Read the model definition and answer for the solid it produces. Units are mm, in the model's axes. Face numbers are marked on the shaded views. Coordinates: 2 decimals unless noted, no trailing zeros. Order: outer loops, then holes, each group sorted by start corner. A loop starts at its lowest first (then second) coordinate and runs counter-clockwise, first axis right, second up. Notation, with made-up numbers: (-25, 45) -> (-15, 45) arc R28 ccw to (-15, 71) -> close; hole circle Ø3 at (14, -8.5). An arc over 180 degrees is marked (long way). Use CSV: the item, a comma, the result in double quotes.
```python
from build123d import *

# Parameters (mm, degrees)
SKETCH1_R           = 32
SKETCH1_R_2         = 2
SKETCH1_R_3         = 4
BOSS_EXTRUDE1_DEPTH = 3
FILLET1_R           = 50


with BuildPart() as part:
    # Sketch1 → Boss-Extrude1 (new body)
    with BuildSketch(Plane(origin=(0, 0, 0), x_dir=(1, 0, 0), z_dir=(0, 1, 0))):
        with Locations(Location((0, 0, 0), (0, 0, 270))):
            Circle(SKETCH1_R)
        with Locations(Location((0, 10, 0), (0, 0, 270))):
            Circle(SKETCH1_R_2, mode=Mode.SUBTRACT)
        with Locations(Location((0, -5, 0), (0, 0, 270))):
            Circle(SKETCH1_R_2, mode=Mode.SUBTRACT)
        with Locations(Location((0, 21.162401824, 0), (0, 0, 270))):
            Circle(SKETCH1_R_3, mode=Mode.SUBTRACT)
        with Locations(Location((16.54543199, 13.19454172, 0), (0, 0, 270))):
            Circle(SKETCH1_R_3, mode=Mode.SUBTRACT)
        with Locations(Location((20.631816227, -4.709077419, 0), (0, 0, 270))):
            Circle(SKETCH1_R_3, mode=Mode.SUBTRACT)
        with Locations(Location((9.182022032, -19.066665213, 0), (0, 0, 270))):
            Circle(SKETCH1_R_3, mode=Mode.SUBTRACT)
        with Locations(Location((-9.182022032, -19.066665213, 0), (0, 0, 270))):
            Circle(SKETCH1_R_3, mode=Mode.SUBTRACT)
        with Locations(Location((-20.631816227, -4.709077419, 0), (0, 0, 270))):
            Circle(SKETCH1_R_3, mode=Mode.SUBTRACT)
        with Locations(Location((-16.54543199, 13.19454172, 0), (0, 0, 270))):
            Circle(SKETCH1_R_3, mode=Mode.SUBTRACT)
    extrude(amount=BOSS_EXTRUDE1_DEPTH)

    # Sketch3 → Revolve2 (revolve)
    with BuildSketch(Plane(origin=(0, 0, 0), x_dir=(0, 0, -1), z_dir=(1, 0, 0))):
        Polygon((-32, 3), (-35.959611008, 28), (-34.959611008, 28), (-30.524846679, 0), (-32, 0), align=None)
    revolve(axis=Axis((0, 0, 0), (0, 1, 0)))

    # Sketch5 → Revolve3 (revolve)
    with BuildSketch(Plane(origin=(0, 0, 0), x_dir=(0, 0, -1), z_dir=(1, 0, 0)), mode=Mode.PRIVATE) as revolve3_sk:
        Polygon((-35.959611008, 28), (-45.524656283, 73), (-45.524656283, 73.207911691), (-44.546508683, 73.207911691), (-34.981463407, 28.207911691), (-34.959611008, 28), align=None)
    revolve(revolve3_sk.sketch.rotate(Axis((0, 0, 0), (0, 1, 0)), 180), axis=Axis((0, 0, 0), (0, 1, 0)))

    # Fillet1
    fillet1_edges = [part.edges().sort_by_distance(p)[0] for p in [
        (0, 28.207911691, 34.981463407),
    ]]
    fillet(fillet1_edges, radius=FILLET1_R)


solid = part.part
```
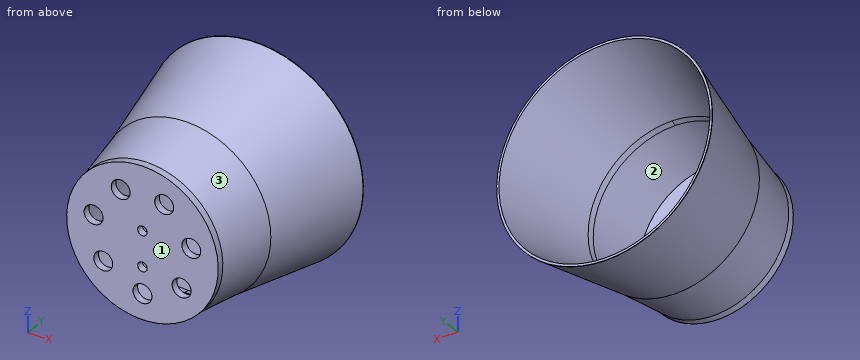
Item 1: Find section A-A, the plane y = 58. Give the vertices of the cut face in (x, z), then the cut area to 3 significant figures.
Return value:
outline,"circle Ø84.67 at (0, 0); hole circle Ø82.63 at (0, 0)"
area,"269 mm^2"
Item 2: Find section C-C, the plane y = 15.5. Give the vertices of the cut face in (x, z), then the cut area to 3 significant figures.
Return value:
outline,"circle Ø67.96 at (0, 0); hole circle Ø65.96 at (0, 0)"
area,"210 mm^2"
Item 3: Each of these flat-tipped pins is pushed along its axis until it touches: P1, Ø4, axis at y = 60, z = -1.5, coming from the +X side; P2, Ø10, axis at x = -17, y = 19.5, coming from the +Z side; P3, Ø13, axis at x = 20.63, z = 4.71, coming from the +Y side. Where does it stop, or does it pass through?
Return value:
P1,"stops at x = 43.17"
P2,"stops at z = 32.65"
P3,"stops at y = 3"
Item 4: Straight lines are drawn through the part: line 1 along X through (y, z) = (2.3, -10); line 2 along X through (y, z) = (70.5, -31); line 3 along X through (y, z) = (10, -3). For each, find the intervals that lie inside material, in ascending order.
Return value:
line 1,"x = -30.4 to -18.95, -14.14 to -2, 2 to 14.14, 18.95 to 30.4"
line 2,"x = -32.61 to -31.18, 31.18 to 32.61"
line 3,"x = -32.97 to -31.97, 31.97 to 32.97"
Item 5: Find section B-B, the plane z = 5. Give the number of separate pieces and of enclosed holes in the cut face, then the cut area to 3 significant figures.
Return value:
separate pieces,"4"
enclosed holes,"0"
area,"273 mm^2"
Item 6: The mould has two halves that part along Z. Classify the marked faces 1, 2 and 3: +Z half, -Z half, draft (parallel to the pull), parting line (faces both ways), or undercut.
Return value:
face 1,"draft"
face 2,"undercut"
face 3,"parting line"
